Check sheet for the modelled part. Datum: model origin and axes. Units: mm. A direction names the side the tool comes from. Round coordinates to 2 decimals unless told otherwise and drop trailing zeros. Order: outer loops, then holes, each group sorted by start corner. A loop starts at its lowest first (then second) coordinate and runs counter-clockwise, first axis right, second up.
(1) Sectioned sample at C-C, the plane z = 67. Enter the section's corners in (x, y).
(2) Sectioned sample at B-B, the plane y = 5.5. Enter the section's corners in (x, z), and give its area (3 significant figures).
(3) Tool access check on faces 4 (the flat face through (-54, 20, -26)), 5 (the flat face through (2, 0, -26)). Record the directions out of +Z, -Z, +X, -X, +Y, -Y that give a thin tool (end or side, any length) a straight path to the whole face; none if there is none.
(4) Depth check by flat-ended pin: pin 1 (5 mm diameter, centred on x = -37, y = 7, fed in from +Z); pin 2 (3 mm diameter, centred on y = 10.5, z = -10, fed in from -X); pin 3 (10 mm diameter, centred on x = -58.5, z = 52, fed in from +Y). Enter the tip coordinate at first touch or a pass-through.
(5) Mould release check, pull along Z, two halves, no side actions. Record for faces 1 (the cylindrical face through (1.648, 34.51, 24.946)), 2 (the cylindrical face through (47.69, 47.69, 15.02)), 3 (the flat face through (-22.9, 70, 10.4)): released by +Z, released by -Z, zero draft, split by the parting line, or undercut.
(6) Thickness scan on probe 1 along Z at (x, y) = (0, 40); probe 2 along X at (y, z) = (17.5, 0.5) (3 decimals). Record the ranges inside material, lowest first.
(7) Sectioned sample at D-D, the plane x = 39.5. Enter the section's corners in (y, z), and give its area (3 significant figures).
Autodesk Inventor part; units mm, degrees
ref_plane "YZ Plane" through (0, 0, 0) normal (1, 0, 0) x (0, 1, 0)
ref_plane "XZ Plane" through (0, 0, 0) normal (0, 1, 0) x (-1, 0, 0)
ref_plane "XY Plane" through (0, 0, 0) normal (0, 0, 1) x (1, 0, 0)
sketch "Sketch1" plane through (0, 0, 0) normal (0, 1, 0) x (-1, 0, 0)
  circle A0 centre (0, 0) radius 125
  circle A1 centre (0, 0) radius 25
  dimension "d0" = 250
  dimension "d3" = 50
extrude "Extrusion1" add sketch "Sketch1" along normal blind 20
sketch "Sketch2" plane through (0, 20, 0) normal (0, 1, 0) x (1, 0, 0)
  circle A0 centre (0, 0) radius 25 construction
  circle A1 centre (0, 0) radius 25
  circle A2 centre (0, 0) radius 50
  dimension "d10" = 100
extrude "Extrusion2" add sketch "Sketch2" along normal blind 50
sketch "Sketch3" plane through (0, 20, 0) normal (0, 1, 0) x (1, 0, 0)
  circle A0 centre (0, 0) radius 50 construction
  circle A1 centre (0, 0) radius 125 construction
  circle A2 centre (0, 0) radius 58
  circle A3 centre (0, 0) radius 50 construction
  circle A4 centre (0, 0) radius 50
  dimension "d6" = 8
  dimension "d7" = 116
extrude "Extrusion3" add sketch "Sketch3" along normal blind 6
properties part number "ShaibaNaPatron"
Derived:
1. outline: (-105.53, 0) - (105.53, 0) - (105.53, 20) - (-105.53, 20) - close
2. outline: circle Ø250 at (0, 0); hole circle Ø50 at (0, 0)
2. area: 47,100 mm2
3. face 4: +Y
3. face 5: +Z, -Z, +X, -X, -Y
4. pin 1: stops at z = 120.14
4. pin 2: stops at x = -124.71
4. pin 3: stops at y = 20
5. face 1: undercut
5. face 2: split by the parting line
5. face 3: zero draft
6. probe 1: z = -50 to -25, 25 to 50
6. probe 2: x = -124.999 to -24.995, 24.995 to 124.999
7. outline: (0, -118.59) - (20, -118.59) - (20, -42.47) - (26, -42.47) - (26, -30.66) - (70, -30.66) - (70, 30.66) - (26, 30.66) - (26, 42.47) - (20, 42.47) - (20, 118.59) - (0, 118.59) - close
7. area: 7,950 mm2
